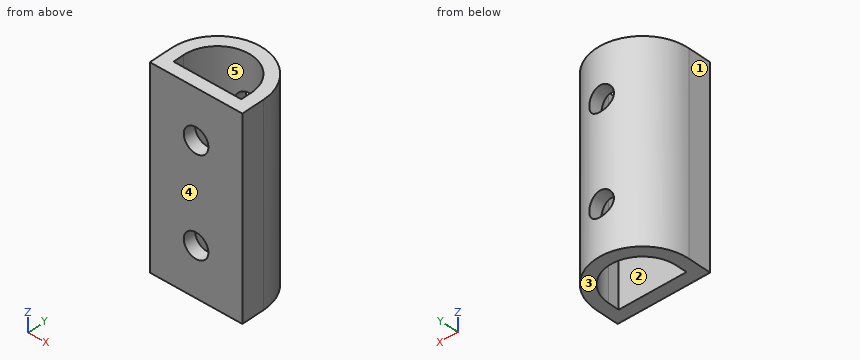
from build123d import *

# Parameters (mm, degrees)
BOSS_EXTRUDE1_DEPTH = 20
CUT_EXTRUDE1_START  = -7.14375
SKETCH2_R           = 1.27
CUT_EXTRUDE1_DEPTH  = 7.14375


with BuildPart() as part:
    # Sketch1 → Boss-Extrude1 (new body)
    with BuildSketch(Plane.XY):
        with BuildLine():
            Line((-4.7625, -2.38125), (4.7625, -2.38125))
            Line((4.7625, -2.38125), (4.7625, 0))
            ThreePointArc((4.7625, 0), (0, 4.7625), (-4.7625, 0))
            Line((-4.7625, 0), (-4.7625, -2.38125))
        make_face()
        with BuildLine():
            Line((-3.4925, -1.11125), (3.4925, -1.11125))
            Line((3.4925, -1.11125), (3.4925, 0))
            ThreePointArc((3.4925, 0), (0, 3.4925), (-3.4925, 0))
            Line((-3.4925, 0), (-3.4925, -1.11125))
        make_face(mode=Mode.SUBTRACT)
    extrude(amount=BOSS_EXTRUDE1_DEPTH)

    # Sketch2 → Cut-Extrude1 (cut)
    with BuildSketch(Plane(origin=(0, -2.38125, 0), x_dir=(-1, 0, 0), z_dir=(0, -1, 0)).offset(CUT_EXTRUDE1_START)):
        with Locations((0, -15.000000033)):
            Circle(SKETCH2_R)
        with Locations((0, -4.999999967)):
            Circle(SKETCH2_R)
    extrude(amount=CUT_EXTRUDE1_DEPTH, mode=Mode.SUBTRACT)


solid = part.part
Could you check a few things on this model? Use its own coordinates, in mm. Face numbers are marked on the shaded views. A direction names the side the tool comes from. Give positions to 0.01 mm unless a question says otherwise; leave off trailing zeros. Order: outer loops, then holes, each group sorted by start corner. A loop starts at its lowest first (then second) coordinate and runs counter-clockwise, first axis right, second up.
Item 1: I'm going to push flat-ended pins straight in: pin 1 (1.5 mm diameter, centred on x = 0, z = 5, fed in from -Y); pin 2 (2 mm diameter, centred on x = 1.5, z = 14.5, fed in from +Y). Where does each tip first touch, or does it pass through?
Item 2: If we mould it in two halves opening along X, with no side actions, what happens to the marked faces 1, 2 and 3? For each: pulls with the +X half, pulls with the -X half, needs draft (parallel to the pull), parting line crosses it, or undercut.
Item 3: If we section it at A-A, the plane x = 0: Write out the boundary of the cut face in (y, z), plus the area to 3 significant figures.
Item 4: If we section it at C-C, the plane z = 15: Write out the boundary of the cut face in (x, y) (1 decimal).
Item 5: For the marked faces 4 and 5, which set-ups out of +Z, -Z, +X, -X, +Y, -Y let a thin tool reach every point of the face, with its end or its side?
Item 6: I need wall thicknesses on line 1 (Z direction, x = 0, y = 4.35); line 2 (X direction, y = -1.55, z = 5); line 3 (X direction, y = 2, z = 4.5). Which ranges of each line are inside material? Lowest first, please.
Item 7: If we section it at B-B, the plane y = -0.5: Write out the boundary of the cut face in (x, z), plus the area to 3 significant figures.
Item 8: If we section it at D-D, the plane x = 3: Write out the boundary of the cut face in (y, z).
Values:
1. pin 1: passes through
1. pin 2: stops at y = 4.71
2. face 1: pulls with the -X half
2. face 2: undercut
2. face 3: needs draft
3. outline: (-2.38, 0) - (-1.11, 0) - (-1.11, 3.73) - (-2.38, 3.73) - close; (-2.38, 6.27) - (-1.11, 6.27) - (-1.11, 13.73) - (-2.38, 13.73) - close; (-2.38, 16.27) - (-1.11, 16.27) - (-1.11, 20) - (-2.38, 20) - close; (3.49, 0) - (4.76, 0) - (4.76, 3.73) - (3.49, 3.73) - close; (3.49, 6.27) - (4.76, 6.27) - (4.76, 13.73) - (3.49, 13.73) - close; (3.49, 16.27) - (4.76, 16.27) - (4.76, 20) - (3.49, 20) - close
3. area: 37.9 mm2
4. outline: (-4.8, -2.4) - (-1.3, -2.4) - (-1.3, -1.1) - (-3.5, -1.1) - (-3.5, 0) arc R3.5 cw to (-1.3, 3.3) - (-1.3, 4.6) arc R4.8 ccw to (-4.8, 0) - close; (1.3, -2.4) - (4.8, -2.4) - (4.8, 0) arc R4.8 ccw to (1.3, 4.6) - (1.3, 3.3) arc R3.5 cw to (3.5, 0) - (3.5, -1.1) - (1.3, -1.1) - close
5. face 4: +Z, -Z, +X, -X, -Y
5. face 5: +Z, -Z
6. line 1: z = 0 to 3.73, 6.27 to 13.73, 16.27 to 20
6. line 2: x = -4.76 to -1.27, 1.27 to 4.76
6. line 3: x = -4.32 to -2.86, 2.86 to 4.32
7. outline: (-4.76, 0) - (-3.49, 0) - (-3.49, 20) - (-4.76, 20) - close; (3.49, 0) - (4.76, 0) - (4.76, 20) - (3.49, 20) - close
7. area: 50.8 mm2
8. outline: (-2.38, 0) - (-1.11, 0) - (-1.11, 20) - (-2.38, 20) - close; (1.79, 0) - (3.7, 0) - (3.7, 20) - (1.79, 20) - close
